Model file for the job. Use its own axes, mm. A direction names the side the tool comes from. Coordinates: 2 decimals unless noted, no trailing zeros. Write each loop counter-clockwise with the first axis right and the second up, starting at its lowest first coordinate (ties: lowest second). Pieces come first, ordered by that corner, then holes. Notation, with made-up numbers: (-10.5, -28.5) - (43.5, -28.5) arc R28 cw to (43.5, 10.5) - close; hole circle Ø8 at (-8.75, 55.25). An arc over 180 degrees is marked (long way). Put each result on its own line as item: value. Start each with the question number.
1. Saw through at B-B, the plane z = 22.25. Write the cut outline in (x, y).
2. Which spindle directions (+Z, -Z, +X, -X, +Y, -Y) get a long thin tool onto all of the face, cutting with end or side? Do faces 4 (the face through (27, 5.08, 22)), 5 (the face through (25, 0, 13)), 6 (the face through (42.349, 6, 4)). Say none if no direction does.
3. Saw through at D-D, the plane y = 6.25. Write the cut outline in (x, z).
4. Drill centre lines: L1, parallel to Z at x = 30.5, y = 3; L2, parallel to Y at x = 20, z = 14; L3, parallel to Z at x = 36, y = 10. Where is each one in solid material? Low to high. Write a range as from..to.
5. Saw through at A-A, the plane x = 28. Write the cut outline in (y, z).
6. Saw through at C-C, the plane y = -2.25. Write the cut outline in (x, z), plus the area to 3 significant figures.
7. Pull direction Y, two halves, no side cores. Call faces 1 (the face through (-7.003, -3.265, 12.522)), 2 (the face through (10.325, 5, 4)), 3 (the face through (26.592, 9.794, 3.812)): released by +Y, released by -Y, zero draft, split by the parting line, or undercut.
8. Drop flat-ended pins along their axis: P1, Ø3, axis at x = 42, z = 6.5, coming from the -Y side; P2, Ø2.5, axis at x = 29.5, y = 7, coming from the -Z side; P3, Ø5, axis at x = 7.5, z = 4.5, coming from the +Y side. Give the stop position or say it passes through.
```python
from build123d import *

# Parameters (mm, degrees)
EXTRUDE_THIN1_DEPTH = 25.4
SKETCH3_W           = 31.939411296
SKETCH3_H           = 2.21446585
BOSS_EXTRUDE1_DEPTH = 2.54
SKETCH4_W           = 31.172865425
SKETCH4_H           = 2.21446585
BOSS_EXTRUDE2_DEPTH = 2.54
BOSS_EXTRUDE3_DEPTH = 2.286
SKETCH10_R          = 1.491946279
CUT_EXTRUDE1_DEPTH  = 70.737718879


with BuildPart() as part:
    # Sketch2 → Extrude-Thin1 (new body)
    with BuildSketch(Plane.XY):
        Polygon((-13.812130674, -6.440702309), (0, 0), (50.8, 0), (64.612130674, -6.440702309), (65.685581059, -4.13868053), (51.363104443, 2.54), (-0.563104443, 2.54), (-14.885581059, -4.13868053), align=None)
    extrude(amount=EXTRUDE_THIN1_DEPTH)

    # Sketch3 → Boss-Extrude1 (add)
    with BuildSketch(Plane(origin=(0, 2.54, 0), x_dir=(1, 0, 0), z_dir=(0, 1, 0))):
        with Locations((26.294303516, -3.760480959)):
            Rectangle(SKETCH3_W, SKETCH3_H)
    extrude(amount=BOSS_EXTRUDE1_DEPTH)

    # Sketch4 → Boss-Extrude2 (add)
    with BuildSketch(Plane(origin=(0, 2.54, 0), x_dir=(1, 0, 0), z_dir=(0, 1, 0))):
        with Locations((26.762748216, -22.000859373)):
            Rectangle(SKETCH4_W, SKETCH4_H)
    extrude(amount=BOSS_EXTRUDE2_DEPTH)

    # Sketch6 → Boss-Extrude3 (add)
    with BuildSketch(Plane(origin=(0, 0, 2.653248034), x_dir=(-1, 0, 0), z_dir=(0, 0, -1))):
        Polygon((-42.349180928, 5.08), (-42.349180928, 7.62), (-35.961730939, 11.406642995), (-16.883255925, 11.406642995), (-10.324597868, 7.62), (-10.324597868, 5.08), align=None)
    extrude(amount=-BOSS_EXTRUDE3_DEPTH)

    # Sketch10 → Cut-Extrude1 (cut, through all)
    with BuildSketch(Plane.XY.offset(4.939248034)):
        with Locations((25.789671125, 8.535532201)):
            Circle(SKETCH10_R)
    extrude(amount=-CUT_EXTRUDE1_DEPTH, mode=Mode.SUBTRACT)


solid = part.part
```
Final values:
1. outline: (-14.89, -4.14) - (-13.81, -6.44) - (0, 0) - (50.8, 0) - (64.61, -6.44) - (65.69, -4.14) - (51.36, 2.54) - (42.35, 2.54) - (42.35, 5.08) - (11.18, 5.08) - (11.18, 2.54) - (-0.56, 2.54) - close
2. face 4: +Z, +X, -X, +Y
2. face 5: +Z, -Z, -Y
2. face 6: +Z, -Z, +X, +Y
3. outline: (10.32, 2.65) - (42.35, 2.65) - (42.35, 4.94) - (10.32, 4.94) - close
4. L1: z = 2.65..4.87, 20.89..23.11
4. L2: y = 0..2.54
4. L3: z = 2.65..4.94
5. outline: (0, 0) - (2.54, 0) - (2.54, 2.65) - (11.41, 2.65) - (11.41, 4.94) - (5.08, 4.94) - (5.08, 4.87) - (2.54, 4.87) - (2.54, 20.89) - (5.08, 20.89) - (5.08, 23.11) - (2.54, 23.11) - (2.54, 25.4) - (0, 25.4) - close
6. outline: (-10.84, 0) - (-4.83, 0) - (-4.83, 25.4) - (-10.84, 25.4) - close; (55.63, 0) - (61.64, 0) - (61.64, 25.4) - (55.63, 25.4) - close
6. area: 305 mm²
7. face 1: released by -Y
7. face 2: zero draft
7. face 3: undercut
8. P1: stops at y = 0
8. P2: stops at z = 2.65
8. P3: stops at y = 2.54
